Geometry: see drawing. Coordinates: mm, zero at the bounding-box minimum. Coordinates: 2 decimals unless noted, no trailing zeros. Loops run counter-clockwise (first coordinate to the right, second up) from the corner with the lowest first, then second, coordinate; pieces in that order, holes last.
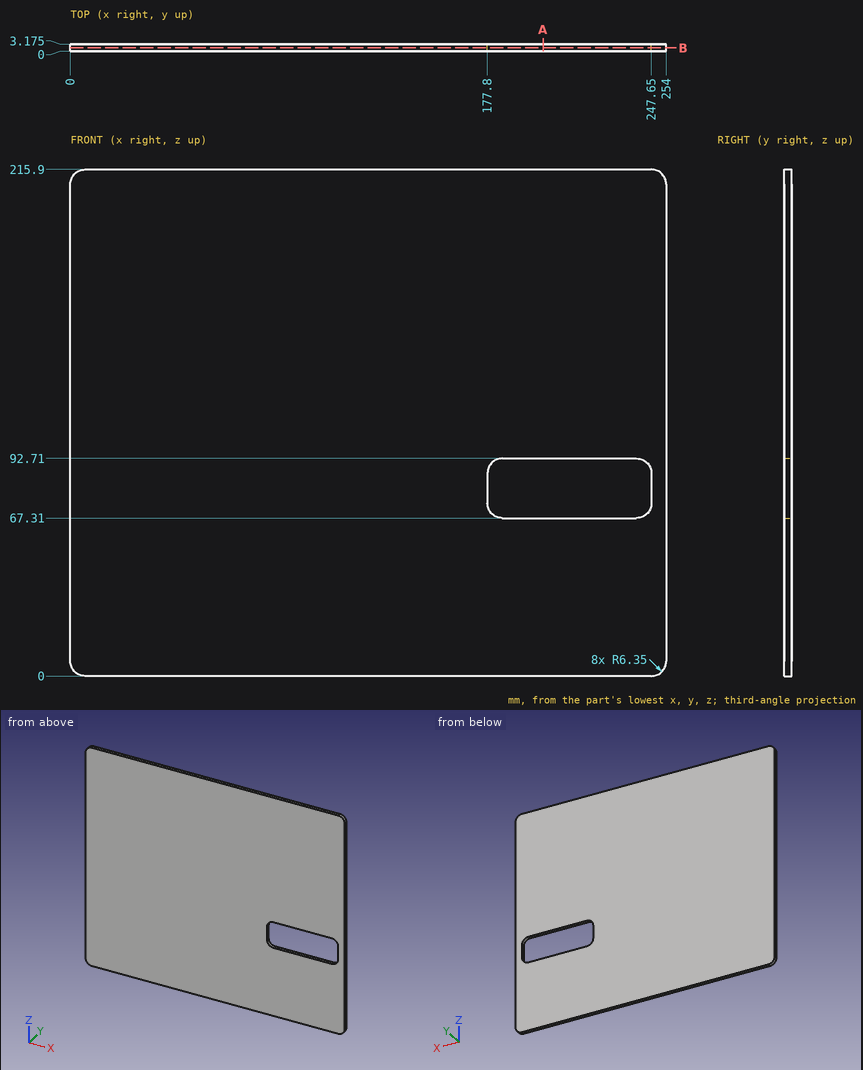
Item 1: Section query B-B (y = 1.5). Output: boundary loops of the cut face in (x, z).
Result:
outline: (0, 6.35) arc R6.35 ccw to (6.35, 0) - (247.65, 0) arc R6.35 ccw to (254, 6.35) - (254, 209.55) arc R6.35 ccw to (247.65, 215.9) - (6.35, 215.9) arc R6.35 ccw to (0, 209.55) - close; hole (177.8, 73.66) arc R6.35 ccw to (184.15, 67.31) - (241.3, 67.31) arc R6.35 ccw to (247.65, 73.66) - (247.65, 86.36) arc R6.35 ccw to (241.3, 92.71) - (184.15, 92.71) arc R6.35 ccw to (177.8, 86.36) - close
Item 2: Line query: L1, parallel to X at y = 0.75, z = 79; L2, parallel to Z at x = 183.5, y = 0.15; L3, parallel to Z at x = 180.5, y = 3. Output: solid intervals per line, ascending.
Result:
L1: x = 0 to 177.8, 247.65 to 254
L2: z = 0 to 67.34, 92.68 to 215.9
L3: z = 0 to 68.46, 91.56 to 215.9
Item 3: Section query A-A (x = 201.5). Output: boundary loops of the cut face in (y, z) (3 decimals).
Result:
outline: (0, 0) - (3.175, 0) - (3.175, 67.31) - (0, 67.31) - close; (0, 92.71) - (3.175, 92.71) - (3.175, 215.9) - (0, 215.9) - close
